Verification items for the finished model (mm, model axes). A direction names the side the tool comes from. Coordinates: 2 decimals unless noted, no trailing zeros. Order: outer loops, then holes, each group sorted by start corner. A loop starts at its lowest first (then second) coordinate and runs counter-clockwise, first axis right, second up. Notation, with made-up numbers: M -3,-7 L 17,-7 A19 ccw 17,-3 Z; hole C 55,34 d5. An arc over 180 degrees is marked long. Write item = value, one per line.
```python
from build123d import *

# Parameters (mm, degrees)
SKETCH1_W           = 154.7
SKETCH1_H           = 52
BOSS_EXTRUDE1_DEPTH = 16
SKETCH3_R           = 3.5
CUT_EXTRUDE2_DEPTH  = 84.156614289
SKETCH5_W           = 26
SKETCH5_H           = 6
CUT_EXTRUDE4_DEPTH  = 95.567555218


with BuildPart() as part:
    # Sketch1 → Boss-Extrude1 (new body)
    with BuildSketch(Plane(origin=(0, 0, 0), x_dir=(1, 0, 0), z_dir=(0, 1, 0))):
        Rectangle(SKETCH1_W, SKETCH1_H)
    extrude(amount=BOSS_EXTRUDE1_DEPTH)

    # Sketch3 → Cut-Extrude2 (cut, through all)
    with BuildSketch(Plane(origin=(0, 16, 0), x_dir=(1, 0, 0), z_dir=(0, 1, 0))):
        with Locations(Location((-69.435638509, 18, 0), (0, 0, 270))):
            Circle(SKETCH3_R)
        with Locations(Location((-33.435638509, 18, 0), (0, 0, 270))):
            Circle(SKETCH3_R)
        with Locations(Location((-33.435638509, -18, 0), (0, 0, 270))):
            Circle(SKETCH3_R)
        with Locations(Location((-69.435638509, -18, 0), (0, 0, 270))):
            Circle(SKETCH3_R)
    cut_extrude2 = extrude(amount=-CUT_EXTRUDE2_DEPTH, mode=Mode.SUBTRACT)

    # Mirror1: Cut-Extrude2 across plane
    add(cut_extrude2.mirror(Plane.ZY), mode=Mode.SUBTRACT)

    # Sketch5 → Cut-Extrude4 (cut, through all)
    with BuildSketch(Plane.XY.offset(26)):
        with Locations((-51.435638509, 13)):
            Rectangle(SKETCH5_W, SKETCH5_H)
    cut_extrude4 = extrude(amount=-CUT_EXTRUDE4_DEPTH, mode=Mode.SUBTRACT)

    # Mirror2: Cut-Extrude4 across plane
    add(cut_extrude4.mirror(Plane.ZY), mode=Mode.SUBTRACT)


solid = part.part
```
Item 1: Sectioned sample at A-A, the plane z = 18. Enter the section's corners in (x, y).
Report:
outline = M -77.35,0 L -72.94,0 L -72.94,16 L -77.35,16 Z; M -65.94,0 L -36.94,0 L -36.94,16 L -38.44,16 L -38.44,10 L -64.44,10 L -64.44,16 L -65.94,16 Z; M -29.94,0 L 29.94,0 L 29.94,16 L -29.94,16 Z; M 36.94,0 L 65.94,0 L 65.94,16 L 64.44,16 L 64.44,10 L 38.44,10 L 38.44,16 L 36.94,16 Z; M 72.94,0 L 77.35,0 L 77.35,16 L 72.94,16 Z
Item 2: Sectioned sample at D-D, the plane z = 1. Enter the section's corners in (x, y).
Report:
outline = M -77.35,0 L 77.35,0 L 77.35,16 L 64.44,16 L 64.44,10 L 38.44,10 L 38.44,16 L -38.44,16 L -38.44,10 L -64.44,10 L -64.44,16 L -77.35,16 Z
Item 3: Sectioned sample at B-B, the plane x = -31.5. Enter the section's corners in (y, z), then the cut area to 3 significant figures.
Report:
outline = M 0,-26 L 16,-26 L 16,-20.92 L 0,-20.92 Z; M 0,-15.08 L 16,-15.08 L 16,15.08 L 0,15.08 Z; M 0,20.92 L 16,20.92 L 16,26 L 0,26 Z
area = 645 mm^2
Item 4: Gauge pin test, flat end, axial feed: pin 1 (11 mm diameter, centred on x = -69.44, z = -18, fed in from +Y). Record the tip position at first contact, or that the pin passes through.
Report:
pin_1 = 16
Item 5: Sectioned sample at C-C, the plane y = 7.5. Give the number of separate pieces and of enclosed holes in the cut face, then the cut area to 3 significant figures.
Report:
separate_pieces = 1
enclosed_holes = 8
area = 7,740 mm^2
Item 6: Scan lines: L1, parallel to X at y = 8, z = 18; L2, parallel to X at y = 11, z = 2.5; L3, parallel to Y at x = 51.5, z = -23. Record each from-to range of solid material in increasing order. Write a range as from..to.
Report:
L1 = -77.35..-72.94, -65.94..-36.94, -29.94..29.94, 36.94..65.94, 72.94..77.35
L2 = -77.35..-64.44, -38.44..38.44, 64.44..77.35
L3 = 0..10
Item 7: Tool access check on faces 1 (the flat face through (77.35, 8, 0)), 2 (the flat face through (-38.436, 13, 0)). Record the directions out of +Z, -Z, +X, -X, +Y, -Y that give a thin tool (end or side, any length) a straight path to the whole face; none if there is none.
Report:
face_1 = +Z, -Z, +X, +Y, -Y
face_2 = +Z, -Z, +Y
Item 8: Release check for a two-part mould opening along X. For faces 3 (the flat face through (-77.35, 8, 0)), 4 (the flat face through (-1, 0, 0)), 5 (the cylindrical face through (-29.965, 8.112, -18.456)) record: pulls with the +X half, pulls with the -X half, needs draft (parallel to the pull), parting line crosses it, or undercut.
Report:
face_3 = pulls with the -X half
face_4 = needs draft
face_5 = undercut
